```python
from build123d import *

# Parameters (mm, degrees)
CYLINDER014005855_R     = 7
CYLINDER014005855_DEPTH = 1
TUBE004_R               = 8
TUBE004_R_2             = 4.2
TUBE004_DEPTH           = 4


with BuildPart() as obj1:
    # Cylinder014005855 → Cylinder014005855 (new body)
    with BuildSketch(Plane.XY):
        Circle(CYLINDER014005855_R)
    extrude(amount=CYLINDER014005855_DEPTH)


with BuildPart() as ring:
    # Tube004 → Tube004 (new body)
    with BuildSketch(Plane.XY):
        Circle(TUBE004_R)
        Circle(TUBE004_R_2, mode=Mode.SUBTRACT)
    extrude(amount=TUBE004_DEPTH)

    # Cut009003003007: cut obj1
    add(obj1.part, mode=Mode.SUBTRACT)


solid = ring.part
```
Input: part model. Units: mm. Frame: model coordinates. A direction names the side the tool comes from. Give positions to 0.01 mm unless a question says otherwise; leave off trailing zeros. Order: outer loops, then holes, each group sorted by start corner. A loop starts at its lowest first (then second) coordinate and runs counter-clockwise, first axis right, second up. Notation, with made-up numbers: M 20.5,65 L 69.5,65 A25 ccw 69.5,96 Z; hole C 87.5,-9.5 d4. An arc over 180 degrees is marked long. Return JSON: item names as keys, results as strings.
Item 1: Access query for faces 1 (the cylindrical face through (4.006, 1.262, 2.479)), 2 (the cylindrical face through (6.466, -2.681, 0.493)). Directions: +Z, -Z, +X, -X, +Y, -Y. A direction counts if a zero-diameter tool reaches every point of the face in a straight line with its end or side. Return the directions, or none.
Solutions:
{"face 1": "+Z, -Z", "face 2": "-Z"}
Item 2: Cut plane D-D (y = 6.25). Return loops of the section in (x, z), then the cut area to 3 significant figures.
Solutions:
{"outline": "M -4.99,0 L -3.15,0 L -3.15,1 L 3.15,1 L 3.15,0 L 4.99,0 L 4.99,4 L -4.99,4 Z", "area": "33.6 mm^2"}
Item 3: First-contact query: P1, Ø3, axis at x = -2, y = 4, coming from the -Z side; P2, Ø1.5, axis at y = -5, z = 3.5, coming from the -X side. Flat tips, straight axial feed; report the tip coordinate or a pass-through.
Solutions:
{"P1": "z = 1", "P2": "x = -6.78"}
Item 4: Pull-direction query (Y, two-part tool) for faces 3 (the flat face through (0, -5, 1)), 4 (the cylindrical face through (-1.73, -7.81, 1.97)), 5 (the flat face through (4, -6, 0)); classes: +Y half, -Y half, draft (parallel to the pull), parting line (faces both ways), or undercut.
Solutions:
{"face 3": "undercut", "face 4": "parting line", "face 5": "draft"}
Item 5: Cut plane A-A (y = 0). Return loops of the section in (x, z).
Solutions:
{"outline": "M -8,0 L -7,0 L -7,1 L -4.2,1 L -4.2,4 L -8,4 Z; M 4.2,1 L 7,1 L 7,0 L 8,0 L 8,4 L 4.2,4 Z"}
Item 6: Cut plane C-C (z = 1.35). Return loops of the section in (x, y).
Solutions:
{"outline": "C 0,0 d16; hole C 0,0 d8.4"}
Item 7: Ray query, probe 1 along Y at (x, z) = (0, 0.9); probe 2 along X at (y, z) = (-2, 1.4); probe 3 along Z at (x, y) = (6.75, -1). Return the intervals inside material, ascending.
Solutions:
{"probe 1": "-8 to -7, 7 to 8", "probe 2": "-7.75 to -3.69, 3.69 to 7.75", "probe 3": "1 to 4"}
